Build history of the part. All positions in model axes, mm. Face numbers are marked on the shaded views. A direction names the side the tool comes from. Round coordinates to 2 decimals unless told otherwise and drop trailing zeros. Write each loop counter-clockwise with the first axis right and the second up, starting at its lowest first coordinate (ties: lowest second). Pieces come first, ordered by that corner, then holes. Notation, with made-up numbers: (67, 5) - (123, 5) arc R16 ccw to (123, 23) - close; hole circle Ø6 at (-3, 0.5). An arc over 180 degrees is marked (long way). Answer as a JSON object with one key per item and string values. Group by question number.
Item 1: Slice it at A-A, the plane z = -4.75. List the corners of the cut face in (x, y), then the cut area to 3 significant figures.
Item 2: Two-plate mould, pull along X, no slides. Class the marked faces 1, 2 and 3: +X half, -X half, draft (parallel to the pull), parting line (faces both ways), or undercut.
Item 3: Probe line 1 (X direction, y = 0, z = -11); line 2 (X direction, y = 0, z = -2.5); line 3 (Z direction, x = 2.75, y = 2.5). List the from-to ranges inside material, lowest first. Write a range as from..to.
Item 4: Flat gauge pins, fed straight in: pin 1 (6.5 mm diameter, centred on x = 0, y = 0, fed in from +Z); pin 2 (4 mm diameter, centred on y = 3, z = -11, fed in from +X); pin 3 (3 mm diameter, centred on x = 3, z = -5.5, fed in from +Y); pin 4 (5 mm diameter, centred on x = 5, y = -1.5, fed in from -Z). Where does each tip first touch, or does it go through?
Item 5: Which spindle directions (+Z, -Z, +X, -X, +Y, -Y) get a long thin tool onto all of the face, cutting with end or side? Do the marked faces 4, 5, 6 and 7. Say none if no direction does.
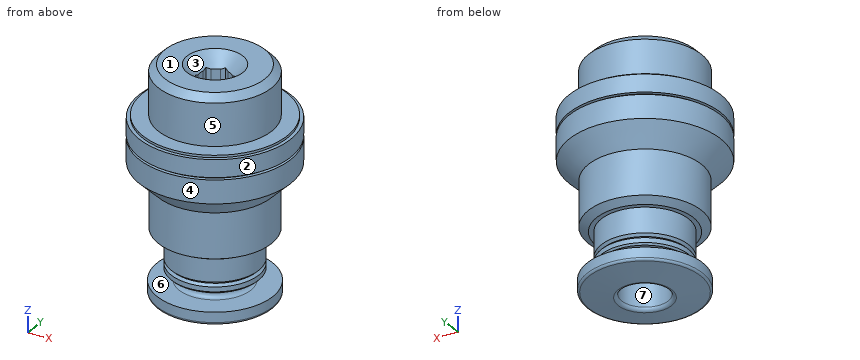
Autodesk Inventor part; units mm, degrees
ref_plane "ANBAU_XY" through (0, 0, 0) normal (0, 0, -1) x (1, 0, 0)
ref_plane "ANBAU_YZ" through (0, 0, 0) normal (1, 0, 0) x (0, -1, 0)
ref_plane "ANBAU_ZX" through (0, 0, 0) normal (0, -1, 0) x (0, 0, -1)
sketch "Sketch_4" plane through (0, 0, 0) normal (1, 0, 0) x (0, 1, 0)
  line L0 (0, -15.3) -> (0, -1.9)
  line L1 (0, -1.9) -> (4.85, -1.9)
  line L2 (4.85, -1.9) -> (4.85, -9.3959)
  line L3 (4.85, -9.3959) -> (4.15, -9.8)
  line L4 (4.15, -9.8) -> (3.75, -9.8)
  line L5 (3.75, -9.8) -> (3.75, -11.95)
  line L6 (3.75, -11.95) -> (3.55, -12.15)
  line L7 (3.55, -12.15) -> (3.75, -12.35)
  line L8 (3.75, -12.35) -> (3.75, -12.7586)
  line L9 (3.75, -12.7586) -> (3.6086, -12.9)
  line L10 (3.6086, -12.9) -> (2.7, -12.9)
  line L11 (2.7, -12.9) -> (2.7, -13.425)
  arc A0 (2.7, -13.425) -> (3.075, -13.8) centre (3.075, -13.425) ccw
  line L12 (3.075, -13.8) -> (4.95, -13.8)
  line L13 (4.95, -13.8) -> (4.95, -14.6649)
  arc A1 (4.7847, -14.8619) -> (4.95, -14.6649) centre (4.75, -14.6649) ccw
  line L14 (4.7847, -14.8619) -> (2.3, -15.3)
  line L15 (2.3, -15.3) -> (0, -15.3)
  line L16 (0, -15.3) -> (0, -1.9)
revolve "Revolution1" add sketch "Sketch_4" angle 360 about axis through (0, 0, -15.3) along (0, 0, -1)
sketch "Sketch_1" plane through (0, 0, 0) normal (1, 0, 0) x (0, 1, 0)
  line L0 (0, -10.4) -> (0, -1.9)
  line L1 (0, -1.9) -> (6.5, -1.9)
  line L2 (6.5, -1.9) -> (6.5, -3.9)
  line L3 (6.5, -3.9) -> (0, -10.4)
  line L4 (0, -10.4) -> (0, -1.9)
revolve "Revolution2" add sketch "Sketch_1" angle 360 about axis through (0, 0, -10.4) along (0, 0, -1)
sketch "Sketch_5" plane through (0, 0, 0) normal (1, 0, 0) x (0, 1, 0)
  line L0 (0, -1.9) -> (0, 4.2)
  line L1 (0, 4.2) -> (4.283, 4.2)
  line L2 (4.283, 4.2) -> (4.864, 3.619)
  line L3 (4.864, 3.619) -> (4.864, 0)
  line L4 (4.864, 0) -> (6.2, 0)
  line L5 (6.2, 0) -> (6.2, -0.2)
  line L6 (6.2, -0.2) -> (6.5, -0.2)
  line L7 (6.5, -0.2) -> (6.5, -1.7)
  line L8 (6.5, -1.7) -> (6.2, -1.7)
  line L9 (6.2, -1.7) -> (6.2, -1.9)
  line L10 (6.2, -1.9) -> (0, -1.9)
  line L11 (0, -1.9) -> (0, 4.2)
revolve "Revolution3" add sketch "Sketch_5" angle 360 about axis through (0, 0, -1.9) along (0, 0, -1)
thread "Thread1"
sketch "Sketch_6" plane through (0, 0, 0) normal (1, 0, 0) x (0, 1, 0)
  line L0 (0, -15.3) -> (0, 4.2)
  line L1 (0, 4.2) -> (2.4, 4.2)
  line L2 (2.4, 4.2) -> (1.3, 3.1)
  line L3 (1.3, 3.1) -> (1.3, -0.4)
  line L4 (1.3, -0.4) -> (2, -0.4)
  line L5 (2, -0.4) -> (2, -15)
  arc A0 (2, -15) -> (2.3, -15.3) centre (2.3, -15) ccw
  line L6 (2.3, -15.3) -> (0, -15.3)
  line L7 (0, -15.3) -> (0, 4.2)
revolve "Revolution4" cut sketch "Sketch_6" angle 360 about axis through (0, 0, -15.3) along (0, 0, -1)
sketch "Sketch_7" plane through (0, 0, 4.2) normal (0, 0, 1) x (1, 0, 0)
  line L0 (-1.25, -0.7217) -> (0, -1.4434)
  line L1 (0, -1.4434) -> (1.25, -0.7217)
  line L2 (1.25, -0.7217) -> (1.25, 0.7217)
  line L3 (1.25, 0.7217) -> (0, 1.4434)
  line L4 (0, 1.4434) -> (-1.25, 0.7217)
  line L5 (-1.25, 0.7217) -> (-1.25, -0.7217)
extrude "Extrusion1" cut sketch "Sketch_7" against normal blind 4.6
ref_plane "ANBAU_XY" through (0, 0, 0) normal (0, 0, -1) x (1, 0, 0)
ref_plane "ANBAU_YZ" through (0, 0, 0) normal (1, 0, 0) x (0, -1, 0)
ref_plane "ANBAU_ZX" through (0, 0, 0) normal (0, -1, 0) x (0, 0, -1)
ref_plane "ANBAU_STD_XY" through (0, 0, 0) normal (0, 0, -1) x (1, 0, 0)
ref_plane "ANBAU_STD_YZ" through (0, 0, 0) normal (1, 0, 0) x (0, -1, 0)
ref_plane "ANBAU_STD_ZX" through (0, 0, 0) normal (0, -1, 0) x (0, 0, -1)
ref_plane "CP_XY" through (0, 0, -15.3) normal (0, 0, -1) x (1, 0, 0)
ref_plane "CP_YZ" through (0, 0, -15.3) normal (1, 0, 0) x (0, -1, 0)
ref_plane "CP_ZX" through (0, 0, -15.3) normal (0, -1, 0) x (0, 0, -1)
ref_plane "CPV_XY" through (0, 0, 0) normal (0, 0, -1) x (1, 0, 0)
ref_plane "CPV_YZ" through (0, 0, 0) normal (1, 0, 0) x (0, -1, 0)
ref_plane "CPV_ZX" through (0, 0, 0) normal (0, -1, 0) x (0, 0, -1)
ref_plane "CPV_ANBAU_XY" through (0, 0, 0) normal (0, 0, -1) x (1, 0, 0)
ref_plane "CPV_ANBAU_YZ" through (0, 0, 0) normal (1, 0, 0) x (0, -1, 0)
ref_plane "CPV_ANBAU_ZX" through (0, 0, 0) normal (0, -1, 0) x (0, 0, -1)
ref_plane "FDT_SCHLAUCH_XY" through (0, 0, -0.4) normal (0, 0, -1) x (1, 0, 0)
ref_plane "FDT_SCHLAUCH_YZ" through (0, 0, -0.4) normal (1, 0, 0) x (0, -1, 0)
ref_plane "FDT_SCHLAUCH_ZX" through (0, 0, -0.4) normal (0, -1, 0) x (0, 0, -1)
properties part number "186106 QS-G1/8-4-I"
Geometry says:
{
 "1": {"outline": "circle Ø11.3 at (0, 0); hole circle Ø4 at (0, 0)", "area": "87.7 mm^2"},
 "2": {"face 1": "draft", "face 2": "parting line", "face 3": "undercut"},
 "3": {"line 1": "x = -3.75..-2, 2..3.75", "line 2": "x = -6.5..-2, 2..6.5", "line 3": "z = -15.05..-13.8, -12.79..-12.32, -11.98..4.2"},
 "4": {"pin 1": "stops at z = 4.2", "pin 2": "stops at x = 4.5", "pin 3": "stops at y = 5.8", "pin 4": "stops at z = -15.23"},
 "5": {"face 4": "+Z, -Z", "face 5": "+Z", "face 6": "none", "face 7": "-Z"}
}
